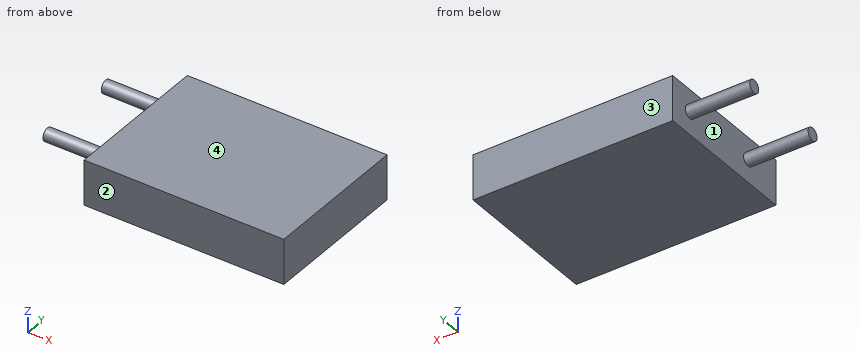
from build123d import *

# Parameters (mm, degrees)
SKETCH_W     = 31
SKETCH_H     = 23
PAD_DEPTH    = 3.5
SKETCH001_R  = 1
PAD001_DEPTH = 10


with BuildPart() as part:
    # Sketch → Pad (new body, symmetric)
    with BuildSketch(Plane.XY):
        Rectangle(SKETCH_W, SKETCH_H)
    extrude(amount=PAD_DEPTH, both=True)

    # Sketch001 (on Face4 of Pad) → Pad001 (join)
    with BuildSketch(Plane(origin=(-15.5, 0, 0), x_dir=(0, -1, 0), z_dir=(-1, 0, 0))):
        with Locations((-7.695191, 0)):
            Circle(SKETCH001_R)
        with Locations((5.304809, 0)):
            Circle(SKETCH001_R)
    extrude(amount=PAD001_DEPTH)


solid = part.part
The model under review builds one solid part; all positions refer to its coordinate system, in mm. Face numbers are marked on the shaded views. Round coordinates to 2 decimals unless told otherwise and drop trailing zeros. Write each loop counter-clockwise with the first axis right and the second up, starting at its lowest first coordinate (ties: lowest second). Pieces come first, ordered by that corner, then holes. Notation, with made-up numbers: M 18,-31.75 L 51,-31.75 A12 cw 51,-15.75 Z; hole C 79,-31 d6. An arc over 180 degrees is marked long. Answer as CSV lines item,"result". Start each with the question number.
Q1. Consider section A-A, the plane x = -18. Give the boundary of the cut face in (y, z).
Q2. Clearance check with a flat-ended pin moving along its axis: P1, Ø3.5, axis at y = 3.5, z = -1, coming from the -X side. State where the tip first meets the part, or that it passes through.
Q3. Consider section D-D, the plane z = -2.5. Give the boundary of the cut face in (x, y), then the cut area to 3 significant figures.
Q4. Consider section B-B, the plane z = 0. Give the boundary of the cut face in (x, y).
Q5. Wall thickness on line 1 along X through (y, z) = (5.75, -2.5); line 2 along Z through (x, y) = (-18, 8.5); line 3 along Z through (x, y) = (-17, 7.25): over which ranges is each line inside the solid? List them lowest first.
Q6. The part is to be moulded in two halves that separate along Y. For the marked faces 1, 2, 3 and 4, say which applies: +Y half, -Y half, draft (parallel to the pull), parting line (faces both ways), or undercut.
Q7. Consider section C-C, the plane y = 1.5. Give the boundary of the cut face in (x, z), then the cut area to 3 significant figures.
Result set:
1,outline,"C -5.3,0 d2; C 7.7,0 d2"
2,P1,"stops at x = -15.5"
3,outline,"M -15.5,-11.5 L 15.5,-11.5 L 15.5,11.5 L -15.5,11.5 Z"
3,area,"713 mm²"
4,outline,"M -25.5,-6.3 L -15.5,-6.3 L -15.5,-11.5 L 15.5,-11.5 L 15.5,11.5 L -15.5,11.5 L -15.5,8.7 L -25.5,8.7 L -25.5,6.7 L -15.5,6.7 L -15.5,-4.3 L -25.5,-4.3 Z"
5,line 1,"x = -15.5 to 15.5"
5,line 2,"z = -0.59 to 0.59"
5,line 3,"z = -0.9 to 0.9"
6,face 1,"undercut"
6,face 2,"-Y half"
6,face 3,"+Y half"
6,face 4,"draft"
7,outline,"M -15.5,-3.5 L 15.5,-3.5 L 15.5,3.5 L -15.5,3.5 Z"
7,area,"217 mm²"
